Autodesk Inventor part; units mm, degrees
ref_plane "Work Plane1" through (8, 0, 0) normal (0, 0, 1) x (1, 0, 0)
ref_plane "YZ Plane" through (0, 0, 0) normal (1, 0, 0) x (0, 1, 0)
ref_plane "XZ Plane" through (0, 0, 0) normal (0, 1, 0) x (-1, 0, 0)
sketch "Sketch1" plane through (0, 0, 0) normal (0, 0, 1) x (1, 0, 0)
  line L0 (0, 0) -> (12.1667, 0)
  line L1 (16, 1.4434) -> (16, 2.5)
  line L2 (16, 2.5) -> (0, 2.5)
  line L3 (16, 1.4434) -> (13, 1.4434)
  line L4 (13, 1.4434) -> (12.1667, 0)
  line L5 (0, -0.5) -> (0, 3)
  line L6 (0, 2.5) -> (0, 0)
  dimension "d0" = 3
  dimension "d1" = 60
  dimension "d2" = 5
  dimension "d3" = 2.8868
  dimension "d5" = 16
revolve "Body" add sketch "Sketch1" angle 360 about axis through (0, 0, 0) along (1, 0, 0)
sketch "Sketch2" plane through (16, 0, 0) normal (1, 0, 0) x (0, 1, 0)
  circle A0 centre (0, 0) radius 1.4434
  line L0 (-0.7217, 1.25) -> (0.7217, 1.25)
  line L1 (0.7217, 1.25) -> (1.4434, 0)
  line L2 (1.4434, 0) -> (0.7217, -1.25)
  line L3 (0.7217, -1.25) -> (-0.7217, -1.25)
  line L4 (-0.7217, -1.25) -> (-1.4434, 0)
  line L5 (-1.4434, 0) -> (-0.7217, 1.25)
  point P0 (0, 0)
  point P1 (0, 0)
extrude "Slot" add sketch "Sketch2" against normal up to next contours L1 A0 | A0 L2 | L0 A0 | A0 L3 | L5 A0 | A0 L4
thread "Thread"
chamfer "Chamfer1" distance 0.4908 angle 45 1 edges at (16, -2.5, 0) measured on face at (10.6667, 2.4676, -0.401)
chamfer "Chamfer2" distance 0.4908 angle 45 1 edges at (0, -2.5, 0) measured on face at (5.1697, 2.4919, -0.2012)
ref_plane "Work Plane1" through (8, 0, 0) normal (0, 0, 1) x (1, 0, 0)
equation "\"d8\" = NLG"
equation "\"d10\" = -0.5 * GD1 + 0.5 * NND"
equation "\"d11\" = FAWI"
equation "\"d34\" = -0.5 * GD1 + 0.5 * NND"
equation "\"d12\" = -0.5 * GD1 + 0.5 * NND"
equation "\"d13\" = FAWI"
equation "\"d35\" = -0.5 * GD1 + 0.5 * NND"
equation "\"d0\" = INTI"
equation "\"d2\" = NND"
equation "\"d3\" = 1.1547 * SW"
equation "\"d5\" = NLG"
equation "\"NND\" = 5"
equation "\"NLG\" = 16"
equation "\"INTI\" = 3"
equation "\"FAWI\" = 45deg"
equation "\"SW\" = 2.5"
equation "\"GD1\" = THREADDIA - 1.2269 * PTC"
equation "\"SPD\" = 3.5"
equation "\"GUL\" = 0.61345 * PTC"
equation "\"TOA\" = 30deg"
equation "\"THREADDIA\" = 5"
equation "\"PTC\" = 0.8"
equation "\"FAWI1\" = 45deg"
equation "\"GAL\" = 0.61345 * PTC"
equation "\"E0\" = 1.155 * SW"
properties part number "DIN 913 - M5 x 16" material "Steel, Mild"
Could you check a few things on this model? Use its own coordinates, in mm. Coordinates: 2 decimals unless noted, no trailing zeros. Write each loop counter-clockwise with the first axis right and the second up, starting at its lowest first coordinate (ties: lowest second). Pieces come first, ordered by that corner, then holes. Notation, with made-up numbers: (-7, 32.5) -> (25, 32.5) arc R9 ccw to (25, 36.5) -> close; hole circle Ø11 at (7, 54). An arc over 180 degrees is marked (long way). One line per question, with ' | ' between items. Start each with the question number.
1. Will these pins go through, and if not, where does the flat tip stop? P1, Ø1, axis at x = 2.5, z = -1, coming from the -Y side; P2, Ø1.5, axis at x = 13, y = -2, coming from the -Z side; P3, Ø1.5, axis at x = 8.5, z = -2, coming from the +Y side.
2. Please list where these lines run through material, in increasing order: line 1 along X through (y, z) = (-0.15, 0.95); line 2 along Z through (x, y) = (7.75, 1.6); line 3 along Y through (x, z) = (6, -2.05).
3. If we section it at A-A (x = 7): Please give me the cut outline in (y, z), and give its area (3 significant figures).
4. Thinking about a two-plate mould opening in Y: for faces 1 (the face through (0, 0, 0)), 2 (the face through (7.89, -0.54, 2.44)), 3 (the face through (14, 0, -1.25)), which applies, pulls with the +Y half, pulls with the -Y half, needs draft (parallel to the pull), parting line crosses it, or undercut?
Return value:
1) P1: stops at y = -2.45 | P2: stops at z = -2.17 | P3: stops at y = 2.17
2) line 1: x = 0 to 12.72 | line 2: z = -1.92 to 1.92 | line 3: y = -1.43 to 1.43
3) outline: circle Ø5 at (0, 0) | area: 19.6 mm²
4) face 1: needs draft | face 2: parting line crosses it | face 3: undercut
